The listing builds one solid part. Answer for the finished solid, in the listing's coordinates (mm). A direction names the side the tool comes from. Give positions to 0.01 mm unless a question says otherwise; leave off trailing zeros. Order: outer loops, then holes, each group sorted by start corner. A loop starts at its lowest first (then second) coordinate and runs counter-clockwise, first axis right, second up. Notation, with made-up numbers: (39.5, 31.5) - (88.5, 31.5) arc R15 ccw to (88.5, 56.5) - close; hole circle Ø1 at (43, 5.5). An arc over 180 degrees is marked (long way). Use a Markdown table: item, result. Add a question column.
1) Straight lines are drawn through the part: line 1 (X direction, y = -12, z = -14); line 2 (X direction, y = -16, z = -33); line 3 (Y direction, x = -19.5, z = -2.5). For each, find the intervals that lie inside material, in ascending order.
2) Find section B-B, the plane y = -17. Determine the outline of the cut face in (x, z).
3) Find section C-C, the plane z = -5. Determine the outline of the cut face in (x, y).
4) Find section A-A, the plane x = -17.5. Determine the outline of the cut face in (y, z).
5) The mould has two halves that part along Y. Classify faces 4 (the face through (3, 0, -21)), 5 (the face through (-2.6, 21.5, -12.2)), 6 (the face through (-16, -3, -2)), 7 (the face through (-16, -13, -2)): released by +Y, released by -Y, zero draft, split by the parting line, or undercut.
6) Flat-ended cylindrical pins translate along their axes: pin 1 (3.5 mm diameter, centred on y = -5, z = -15, fed in from -X); pin 2 (4 mm diameter, centred on y = 1, z = -27, fed in from +X); pin 3 (1.5 mm diameter, centred on x = 4.5, y = -3.5, fed in from +Z). Find the tip coordinate at first contact, or state that the pin passes through.
7) For faces 1 (the face through (-3.5, 0, -19)), 2 (the face through (3, 0, -15)), 3 (the face through (-16, 19, -2)), determine the directions among +Z, -Z, +X, -X, +Y, -Y from which every point of the face is accessible in a straight line to the end or side of a thin tool.
8) Find section D-D, the plane x = -6.5. Determine the outline of the cut face in (y, z), plus the area to 3 significant figures.
from build123d import *

# Parameters (mm, degrees)
P_IDAT_VYSUNUT_M1_DEPTH  = 21.5
P_IDAT_VYSUNUT_M2_DEPTH  = 3
P_IDAT_VYSUNUT_M3_DEPTH  = 3
ODEBRAT_VYSUNUT_M1_DEPTH = 50.550075681
ZAOBLIT1_R               = 2.5
ZAOBLIT2_R               = 0.5


with BuildPart() as part:
    # Skica2 → Přidat vysunutím1 (new, symmetric)
    with BuildSketch(Plane(origin=(0, 0, 0), x_dir=(1, 0, 0), z_dir=(0, 1, 0))):
        Polygon((0, 0), (-26.4, 0), (-26.4, 3.4), (-3.5, 3.4), (-3.5, 36), (0, 36), align=None)
    extrude(amount=P_IDAT_VYSUNUT_M1_DEPTH, both=True)

    # Skica3 → Přidat vysunutím2 (add)
    with BuildSketch(Plane(origin=(0, 0, 0), x_dir=(0, 0, -1), z_dir=(1, 0, 0))):
        with BuildLine():
            Line((16.6, 15.48178046), (16.6, -15.48178046))
            ThreePointArc((16.6, -15.48178046), (18, -15.7), (19.4, -15.48178046))
            Line((19.4, -15.48178046), (19.4, 15.48178046))
            ThreePointArc((19.4, 15.48178046), (18, 15.7), (16.6, 15.48178046))
        make_face()
    extrude(amount=P_IDAT_VYSUNUT_M2_DEPTH)

    # Skica4 → Přidat vysunutím3 (add)
    with BuildSketch(Plane(origin=(3, 0, 0), x_dir=(0, 0, -1), z_dir=(1, 0, 0))):
        with BuildLine():
            Line((13.4, -11.1), (13.4, 11.1))
            ThreePointArc((13.4, 11.1), (18, 15.7), (22.6, 11.1))
            Line((22.6, 11.1), (22.6, -11.1))
            ThreePointArc((22.6, -11.1), (18, -15.7), (13.4, -11.1))
        make_face()
    extrude(amount=P_IDAT_VYSUNUT_M3_DEPTH)

    # Skica5 → Odebrat vysunutím1 (cut, through all)
    with BuildSketch(Plane.XY):
        with BuildLine():
            Line((-14.400164981, -3), (-18.399835019, -3))
            ThreePointArc((-18.399835019, -3), (-21.399835019, 0), (-18.399835019, 3))
            Line((-18.399835019, 3), (-14.400164981, 3))
            ThreePointArc((-14.400164981, 3), (-11.400164981, 0), (-14.400164981, -3))
        make_face()
        with BuildLine():
            Line((-14.400164981, 13), (-18.399835019, 13))
            ThreePointArc((-18.399835019, 13), (-21.399835019, 16), (-18.399835019, 19))
            Line((-18.399835019, 19), (-14.400164981, 19))
            ThreePointArc((-14.400164981, 19), (-11.400164981, 16), (-14.400164981, 13))
        make_face()
        with BuildLine():
            Line((-14.400164981, -19), (-18.399835019, -19))
            ThreePointArc((-18.399835019, -19), (-21.399835019, -16), (-18.399835019, -13))
            Line((-18.399835019, -13), (-14.400164981, -13))
            ThreePointArc((-14.400164981, -13), (-11.400164981, -16), (-14.400164981, -19))
        make_face()
    extrude(amount=-ODEBRAT_VYSUNUT_M1_DEPTH, mode=Mode.SUBTRACT)

    # Zaoblit1
    zaoblit1_edges = [part.edges().sort_by_distance(p)[0] for p in [
        (-26.4, 21.5, -1.7),
        (-26.4, -21.5, -1.7),
        (-1.75, 21.5, -36),
        (-1.75, -21.5, -36),
    ]]
    fillet(zaoblit1_edges, radius=ZAOBLIT1_R)

    # Zaoblit2
    zaoblit2_edges = [part.edges().sort_by_distance(p)[0] for p in [
        (0, 0, 0),
        (-26.4, 0, 0),
        (-26.4, 0, -3.4),
        (-11.95, -21.5, 0),
        (-11.95, 21.5, 0),
        (-25.667766953, 20.767766953, 0),
        (-25.667766953, -20.767766953, 0),
        (-3.5, -21.5, -18.45),
        (-25.667766953, 20.767766953, -3.4),
        (-25.667766953, -20.767766953, -3.4),
        (-3.5, 21.5, -18.45),
        (-3.5, 0, -36),
        (0, 0, -36),
        (-3.5, 20.767766953, -35.267766953),
        (-3.5, -20.767766953, -35.267766953),
        (0, 20.767766953, -35.267766953),
        (0, -20.767766953, -35.267766953),
        (-13.7, 21.5, -3.4),
        (0, 21.5, -16.75),
        (-13.7, -21.5, -3.4),
        (0, -21.5, -16.75),
    ]]
    fillet(zaoblit2_edges, radius=ZAOBLIT2_R)


solid = part.part
The answers:
| question | item | result |
|---|---|---|
| 1 | line 1 | -3.5 to 0, 3 to 6 |
| 1 | line 2 | -3.5 to 0 |
| 1 | line 3 | -21.5 to -18.79, -13.21 to -2.79, 2.79 to 13.21, 18.79 to 21.5 |
| 2 | outline | (-26.4, -2.9) arc R0.5 ccw to (-25.9, -3.4) - (-21.23, -3.4) - (-21.23, 0) - (-25.9, 0) arc R0.5 ccw to (-26.4, -0.5) - close; (-11.57, -3.4) - (-3.5, -3.4) - (-3.5, -35.5) arc R0.5 ccw to (-3, -36) - (-0.5, -36) arc R0.5 ccw to (0, -35.5) - (0, -0.5) arc R0.5 ccw to (-0.5, 0) - (-11.57, 0) - close |
| 3 | outline | (-3.5, -21) arc R0.5 ccw to (-3, -21.5) - (-0.5, -21.5) arc R0.5 ccw to (0, -21) - (0, 21) arc R0.5 ccw to (-0.5, 21.5) - (-3, 21.5) arc R0.5 ccw to (-3.5, 21) - close |
| 4 | outline | (-21.5, -2.9) arc R0.5 ccw to (-21, -3.4) - (-19, -3.4) - (-19, 0) - (-21, 0) arc R0.5 ccw to (-21.5, -0.5) - close; (-13, -3.4) - (-3, -3.4) - (-3, 0) - (-13, 0) - close; (3, -3.4) - (13, -3.4) - (13, 0) - (3, 0) - close; (19, -3.4) - (21, -3.4) arc R0.5 ccw to (21.5, -2.9) - (21.5, -0.5) arc R0.5 ccw to (21, 0) - (19, 0) - close |
| 5 | face 4 | zero draft |
| 5 | face 5 | released by +Y |
| 5 | face 6 | undercut |
| 5 | face 7 | undercut |
| 6 | pin 1 | x = -3.5 |
| 6 | pin 2 | x = 0 |
| 6 | pin 3 | z = -13.4 |
| 7 | face 1 | -Z, -X, +Y, -Y |
| 7 | face 2 | +Z, +Y, -Y |
| 7 | face 3 | +Z, -Z |
| 8 | outline | (-21.5, -2.9) arc R0.5 ccw to (-21, -3.4) - (21, -3.4) arc R0.5 ccw to (21.5, -2.9) - (21.5, -0.5) arc R0.5 ccw to (21, 0) - (-21, 0) arc R0.5 ccw to (-21.5, -0.5) - close |
| 8 | area | 146 mm2 |
